Part model, mm, in its own coordinate system. A direction names the side the tool comes from. Round coordinates to 2 decimals unless told otherwise and drop trailing zeros. Write each loop counter-clockwise with the first axis right and the second up, starting at its lowest first coordinate (ties: lowest second). Pieces come first, ordered by that corner, then holes. Notation, with made-up numbers: (-6.75, -32) -> (51.25, -32) arc R25 cw to (51.25, -17) -> close; hole circle Ø10 at (-7, 9). An arc over 180 degrees is marked (long way). Use CSV: the item, a comma, the result in double quotes. Start each with the question number.
```python
from build123d import *

# Parameters (mm, degrees)
SKETCH_1_W               = 56
SKETCH_1_H               = 50
SKETCH_1_R               = 1.6
EXTRUDE_1_DEPTH          = 7.6
CUT_EXTRUDE_START        = -1.6
SKETCH_2_W               = 50.2
SKETCH_2_H               = 50
SKETCH_2_R               = 1.6
CUT_EXTRUDE_1_DEPTH      = 1.6
CUT_EXTRUDE_START_2      = -4
SKETCH_3_W               = 40.2
SKETCH_3_H               = 38
SKETCH_3_R               = 1.6
SKETCH_3_H_2             = 6
SKETCH_3_W_2             = 5
CUT_EXTRUDE_2_DEPTH      = 4
SKETCH_4_R               = 2.6
SKETCH_4_R_2             = 1.6
EXTRUDE_2_DEPTH          = 4
SKETCH_6_W               = 40.2
SKETCH_6_H               = 2
EXTRUDE_3_DEPTH          = 4
FILLET_2_R               = 2
SKETCH_7_R               = 2.8
CUT_EXTRUDE_3_DEPTH      = 3.2
PATTERN_CIRCULAR_2_COUNT = 4


with BuildPart() as part:
    # 草图1 → 凸台-拉伸1 (new body)
    with BuildSketch(Plane(origin=(0, 0, 0), x_dir=(1, 0, 0), z_dir=(0, 1, 0))):
        Rectangle(SKETCH_1_W, SKETCH_1_H)
        with Locations(Location((-12.5, 12.5, 0), (0, 0, 90))):
            Circle(SKETCH_1_R, mode=Mode.SUBTRACT)
        with Locations(Location((12.5, 12.5, 0), (0, 0, 90))):
            Circle(SKETCH_1_R, mode=Mode.SUBTRACT)
        with Locations(Location((12.5, -12.5, 0), (0, 0, 90))):
            Circle(SKETCH_1_R, mode=Mode.SUBTRACT)
        with Locations(Location((-12.5, -12.5, 0), (0, 0, 90))):
            Circle(SKETCH_1_R, mode=Mode.SUBTRACT)
    extrude(amount=EXTRUDE_1_DEPTH)

    # 草图2 → 切除-拉伸1 (cut)
    with BuildSketch(Plane(origin=(0, 7.6, 0), x_dir=(1, 0, 0), z_dir=(0, 1, 0)).offset(CUT_EXTRUDE_START)):
        Rectangle(SKETCH_2_W, SKETCH_2_H)
        with Locations(Location((-12.5, -12.5, 0), (0, 0, 90))):
            Circle(SKETCH_2_R, mode=Mode.SUBTRACT)
        with Locations(Location((12.5, -12.5, 0), (0, 0, 90))):
            Circle(SKETCH_2_R, mode=Mode.SUBTRACT)
        with Locations(Location((-12.5, 12.5, 0), (0, 0, 90))):
            Circle(SKETCH_2_R, mode=Mode.SUBTRACT)
        with Locations(Location((12.5, 12.5, 0), (0, 0, 90))):
            Circle(SKETCH_2_R, mode=Mode.SUBTRACT)
    extrude(amount=CUT_EXTRUDE_1_DEPTH, mode=Mode.SUBTRACT)

    # 草图3 → 切除-拉伸2 (cut)
    # profile 1 of 5: a face of its own
    with BuildSketch(Plane(origin=(0, 6, 0), x_dir=(1, 0, 0), z_dir=(0, 1, 0)).offset(CUT_EXTRUDE_START_2)):
        Rectangle(SKETCH_3_W, SKETCH_3_H)
        with Locations(Location((-12.5, -12.5, 0), (0, 0, 90))):
            Circle(SKETCH_3_R, mode=Mode.SUBTRACT)
        with Locations(Location((12.5, -12.5, 0), (0, 0, 90))):
            Circle(SKETCH_3_R, mode=Mode.SUBTRACT)
        with Locations(Location((-12.5, 12.5, 0), (0, 0, 90))):
            Circle(SKETCH_3_R, mode=Mode.SUBTRACT)
        with Locations(Location((12.5, 12.5, 0), (0, 0, 90))):
            Circle(SKETCH_3_R, mode=Mode.SUBTRACT)
    # profile 2 of 5: a face of its own
    with BuildSketch(Plane(origin=(0, 6, 0), x_dir=(1, 0, 0), z_dir=(0, 1, 0)).offset(CUT_EXTRUDE_START_2)):
        with Locations((0, 22)):
            Rectangle(SKETCH_3_W, SKETCH_3_H_2)
    # profile 3 of 5: a face of its own
    with BuildSketch(Plane(origin=(0, 6, 0), x_dir=(1, 0, 0), z_dir=(0, 1, 0)).offset(CUT_EXTRUDE_START_2)):
        with Locations((22.6, 0)):
            Rectangle(SKETCH_3_W_2, SKETCH_3_H)
    # profile 4 of 5: a face of its own
    with BuildSketch(Plane(origin=(0, 6, 0), x_dir=(1, 0, 0), z_dir=(0, 1, 0)).offset(CUT_EXTRUDE_START_2)):
        with Locations((-22.6, 0)):
            Rectangle(SKETCH_3_W_2, SKETCH_3_H)
    # profile 5 of 5: a face of its own
    with BuildSketch(Plane(origin=(0, 6, 0), x_dir=(1, 0, 0), z_dir=(0, 1, 0)).offset(CUT_EXTRUDE_START_2)):
        with Locations((0, -22)):
            Rectangle(SKETCH_3_W, SKETCH_3_H_2)
    extrude(amount=CUT_EXTRUDE_2_DEPTH, mode=Mode.SUBTRACT)

    # 草图4 → 凸台-拉伸2 (add)
    # profile 1 of 4: a face of its own
    with BuildSketch(Plane(origin=(0, 2, 0), x_dir=(1, 0, 0), z_dir=(0, 1, 0))):
        with Locations(Location((-12.5, 12.5, 0), (0, 0, 270))):
            Circle(SKETCH_4_R)
        with Locations(Location((-12.5, 12.5, 0), (0, 0, 90))):
            Circle(SKETCH_4_R_2, mode=Mode.SUBTRACT)
    # profile 2 of 4: a face of its own
    with BuildSketch(Plane(origin=(0, 2, 0), x_dir=(1, 0, 0), z_dir=(0, 1, 0))):
        with Locations(Location((12.5, 12.5, 0), (0, 0, 270))):
            Circle(SKETCH_4_R)
        with Locations(Location((12.5, 12.5, 0), (0, 0, 90))):
            Circle(SKETCH_4_R_2, mode=Mode.SUBTRACT)
    # profile 3 of 4: a face of its own
    with BuildSketch(Plane(origin=(0, 2, 0), x_dir=(1, 0, 0), z_dir=(0, 1, 0))):
        with Locations(Location((12.5, -12.5, 0), (0, 0, 270))):
            Circle(SKETCH_4_R)
        with Locations(Location((12.5, -12.5, 0), (0, 0, 90))):
            Circle(SKETCH_4_R_2, mode=Mode.SUBTRACT)
    # profile 4 of 4: a face of its own
    with BuildSketch(Plane(origin=(0, 2, 0), x_dir=(1, 0, 0), z_dir=(0, 1, 0))):
        with Locations(Location((-12.5, -12.5, 0), (0, 0, 270))):
            Circle(SKETCH_4_R)
        with Locations(Location((-12.5, -12.5, 0), (0, 0, 90))):
            Circle(SKETCH_4_R_2, mode=Mode.SUBTRACT)
    extrude(amount=EXTRUDE_2_DEPTH)

    # 草图6 → 凸台-拉伸3 (add)
    with BuildSketch(Plane(origin=(0, 2, 0), x_dir=(1, 0, 0), z_dir=(0, 1, 0))):
        with Locations((0, -24)):
            Rectangle(SKETCH_6_W, SKETCH_6_H)
        with Locations((0, 24)):
            Rectangle(SKETCH_6_W, SKETCH_6_H)
    extrude(amount=EXTRUDE_3_DEPTH)

    # 圆角2
    fillet_2_edges = [part.edges().sort_by_distance(p)[0] for p in [
        (25.1, 4, 19),
        (20.1, 4, 19),
        (20.1, 4, 23),
        (-28, 3.8, -25),
        (-28, 3.8, 25),
        (28, 3.8, 25),
        (28, 3.8, -25),
        (-20.1, 4, 23),
        (-25.1, 4, 19),
        (-20.1, 4, 19),
        (25.1, 4, -19),
        (20.1, 4, -19),
        (20.1, 4, -23),
        (-20.1, 4, -23),
        (-20.1, 4, -19),
        (-25.1, 4, -19),
    ]]
    fillet(fillet_2_edges, radius=FILLET_2_R - 0.0001)  # a hair under: the kernel refuses the full size

    # 草图5 → 旋转1 (revolve)
    with BuildSketch(Plane.XY.offset(12.5), mode=Mode.PRIVATE) as revolve_1_sk:
        Polygon((-9.9, 5), (-7.9, 2), (-9.9, 2), align=None)
    revolve_1 = revolve(revolve_1_sk.sketch.rotate(Axis((-12.5, 6, 12.5), (0, -1, 0)), 270), axis=Axis((-12.5, 6, 12.5), (0, -1, 0)))

    # 草图7 → 切除-拉伸3 (cut)
    with BuildSketch(Plane.XZ):
        with Locations(Location((-12.5, 12.5, 0), (0, 0, 270))):
            Circle(SKETCH_7_R)
    cut_extrude_3 = extrude(amount=-CUT_EXTRUDE_3_DEPTH, mode=Mode.SUBTRACT)

    # 阵列(圆周)2: 旋转1, 切除-拉伸3 ×4 about axis
    pattern_circular_2_axis = Axis((0, 0, 0), (0, 1, 0))
    add([revolve_1.rotate(pattern_circular_2_axis, i * 360 / PATTERN_CIRCULAR_2_COUNT) for i in range(1, PATTERN_CIRCULAR_2_COUNT)])
    add([cut_extrude_3.rotate(pattern_circular_2_axis, i * 360 / PATTERN_CIRCULAR_2_COUNT) for i in range(1, PATTERN_CIRCULAR_2_COUNT)], mode=Mode.SUBTRACT)


solid = part.part
```
1. Which spindle directions (+Z, -Z, +X, -X, +Y, -Y) get a long thin tool onto all of the face, cutting with end or side? Do faces 1 (the flat face through (-25.1, 5, 0)), 2 (the flat face through (-14, 6, 11)), 3 (the cylindrical face through (9.83, 1.58, 11.66)). Say none if no direction does.
2. Pull direction Z, two halves, no side cores. Call faces 4 (the flat face through (-27, 7.6, 0)), 5 (the cylindrical face through (-12.57, 4.58, -10.9)), 6 (the flat face through (0, 3, -25)), 7 (the cylindrical face through (27.4, 3.85, 24.43)): released by +Z, released by -Z, zero draft, split by the parting line, or undercut.
3. Flat gauge pins, fed straight in: pin 1 (8 mm diameter, centred on x = 9.5, z = 5.5, fed in from +Y); pin 2 (9 mm diameter, centred on x = -12.5, z = -12.5, fed in from +Y); pin 3 (3 mm diameter, centred on x = -13, z = 13, fed in from -Y). Where does each tip first touch, or does it go through?
4. Band-saw the part on A-A (y = 6.75). List the corners of the cut face in (x, z).
5. Band-saw the part on D-D (x = -7). List the corners of the cut face in (y, z), then the cut area to 3 significant figures.
6. Band-saw the part on B-B (x = 12.5). Give the number of separate pieces and of enclosed holes in the cut face, then the cut area to 3 significant figures.
7. Drill centre lines: line 1 along Z through (x, y) = (15, 3.5); line 2 along Z through (x, y) = (-12.5, 5.25); line 3 along X through (y, z) = (6.5, 16). Where is each one in solid material? Low to high. Write a range as [from, to].
Answers below:
1,face 1,"+Y"
1,face 2,"+Z, -Z, +Y"
1,face 3,"-Y"
2,face 4,"zero draft"
2,face 5,"undercut"
2,face 6,"released by -Z"
2,face 7,"released by +Z"
3,pin 1,"stops at y = 3.48"
3,pin 2,"stops at y = 6"
3,pin 3,"stops at y = 3.2"
4,outline,"(-28, -23) arc R2 ccw to (-26, -25) -> (-25.1, -25) -> (-25.1, 25) -> (-26, 25) arc R2 ccw to (-28, 23) -> close; (25.1, -25) -> (26, -25) arc R2 ccw to (28, -23) -> (28, 23) arc R2 ccw to (26, 25) -> (25.1, 25) -> close"
5,outline,"(0, -25) -> (6, -25) -> (6, -23) -> (2, -23) -> (2, 23) -> (6, 23) -> (6, 25) -> (0, 25) -> close"
5,area,"116 mm^2"
6,separate pieces,"3"
6,enclosed holes,"0"
6,area,"116 mm^2"
7,line 1,"z = [-25, -23], [-15.09, -9.91], [9.91, 15.09], [23, 25]"
7,line 2,"z = [-25, -23], [-15.1, -14.1], [-10.9, -9.9], [9.9, 10.9], [14.1, 15.1], [23, 25]"
7,line 3,"x = [-28, -25.1], [25.1, 28]"
